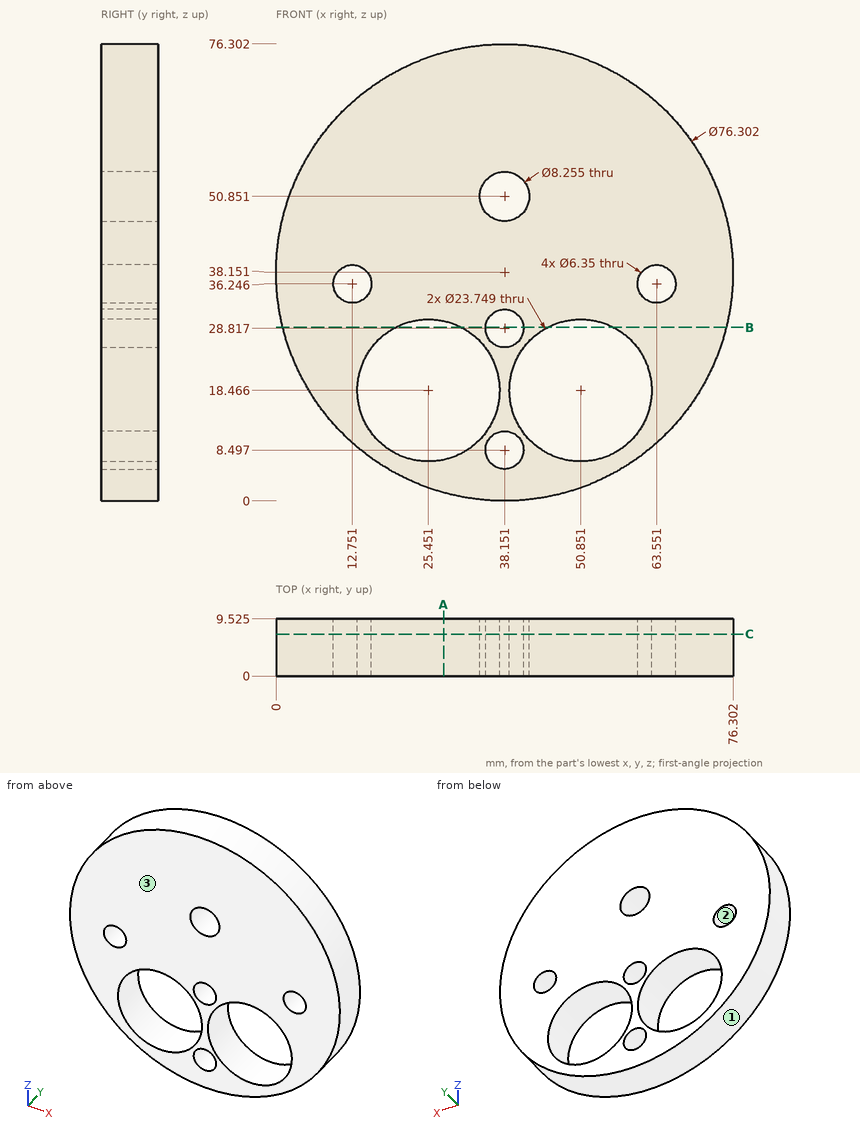
Print and shaded views of the part. All mm, measured from the part's lowest x, y and z. Coordinates: 2 decimals unless noted, no trailing zeros. Order: outer loops, then holes, each group sorted by start corner. A loop starts at its lowest first (then second) coordinate and runs counter-clockwise, first axis right, second up. Notation, with made-up numbers: (81.5, 13) -> (100.5, 13) arc R30 cw to (100.5, 35) -> close; hole circle Ø2 at (-27.5, 8.25). An arc over 180 degrees is marked (long way). Use one line per item in the form item = value. Start each with the question number.
1) Drill centre lines: L1, parallel to X at y = 8.25, z = 15.5; L2, parallel to X at y = 7, z = 26.5 (1 decimal); L3, parallel to X at y = 3, z = 35.5 (1 decimal). Where is each one in solid material? Low to high. Write a range as [from, to].
2) Band-saw the part on C-C on y = 7. State how many separate pieces and enclosed holes the cut face has, then the cut area to 3 significant figures.
3) Pull direction X, two halves, no side cores. Call the marked faces 1, 2 and 3: +X half, -X half, draft (parallel to the pull), parting line (faces both ways), or undercut.
4) Band-saw the part on B-B on z = 29. Give the cut face in (x, y) (1 decimal).
5) Band-saw the part on A-A on x = 28. Give the cut face in (y, z) (1 decimal), then the cut area to 3 significant figures.
6) Drop flat-ended pins along their axis: pin 1 (1.5 mm diameter, centred on x = 63, y = 7.5, fed in from -Z) (1 decimal); pin 2 (10 mm diameter, centred on x = 12.75, z = 36.25, fed in from +Y) (3 decimals); pin 3 (5 mm diameter, centred on y = 2.5, z = 61.5, fed in from -X); pin 4 (1 mm diameter, centred on y = 5.5, z = 19, fed in from -X). Give the stop position or say it passes through.
Entries:
q1.L1 = [7.45, 13.95], [36.95, 39.35], [62.35, 68.85]
q1.L2 = [1.8, 16.7], [34.2, 36], [40.3, 42.1], [59.6, 74.5]
q1.L3 = [0.1, 9.7], [15.8, 60.5], [66.6, 76.2]
q2.separate_pieces = 1
q2.enclosed_holes = 7
q2.area = 3,510 mm2
q3.face_1 = parting line
q3.face_2 = undercut
q3.face_3 = draft
q4.outline = (1.1, 0) -> (20, 0) -> (20, 9.5) -> (1.1, 9.5) -> close; (30.9, 0) -> (35, 0) -> (35, 9.5) -> (30.9, 9.5) -> close; (41.3, 0) -> (45.4, 0) -> (45.4, 9.5) -> (41.3, 9.5) -> close; (56.3, 0) -> (75.2, 0) -> (75.2, 9.5) -> (56.3, 9.5) -> close
q5.outline = (0, 1.4) -> (9.5, 1.4) -> (9.5, 6.9) -> (0, 6.9) -> close; (0, 30.1) -> (9.5, 30.1) -> (9.5, 74.9) -> (0, 74.9) -> close
q5.area = 480 mm2
q6.pin_1 = 8.6
q6.pin_2 = 9.525
q6.pin_3 = 6.2
q6.pin_4 = 4.87
